Work out the finished part from the listing and answer in its coordinate system (mm). Give positions to 0.01 mm unless a question says otherwise; leave off trailing zeros. Loops run counter-clockwise (first coordinate to the right, second up) from the corner with the lowest first, then second, coordinate; pieces in that order, holes last. Notation, with made-up numbers: (23, 85) - (63, 85) arc R14 cw to (63, 111) - close; hole circle Ø11 at (-2, -35.75). An arc over 180 degrees is marked (long way). One line per item, written item: value.
from build123d import *

# Parameters (mm, degrees)
SKETCH_3_W          = 213
SKETCH_3_H          = 65.8
SKETCH_3_R          = 3
EXTRUDE_2_DEPTH     = 5
SKETCH_4_R          = 1.5
CUT_EXTRUDE_1_DEPTH = 5
SKETCH_5_R          = 1.5
CUT_EXTRUDE_2_DEPTH = 5
SKETCH_6_R          = 3
CUT_EXTRUDE_3_DEPTH = 10


with BuildPart() as part:
    # Sketch 3 → Extrude 2 (new body)
    with BuildSketch(Plane.XY):
        Rectangle(SKETCH_3_W, SKETCH_3_H)
        Circle(SKETCH_3_R, mode=Mode.SUBTRACT)
    extrude(amount=EXTRUDE_2_DEPTH)

    # Sketch 4 → Cut-Extrude 1 (cut)
    with BuildSketch(Plane.XY.offset(5)):
        with Locations((60, 12.1)):
            Circle(SKETCH_4_R)
        with Locations((60, -17.9)):
            Circle(SKETCH_4_R)
        with Locations(Location((-60, -17.9, 0), (0, 0, 180))):
            Circle(SKETCH_4_R)
        with Locations(Location((-60, 12.1, 0), (0, 0, 180))):
            Circle(SKETCH_4_R)
    extrude(amount=-CUT_EXTRUDE_1_DEPTH, mode=Mode.SUBTRACT)

    # Sketch 5 → Cut-Extrude 2 (cut)
    with BuildSketch(Plane.XY.offset(5)):
        with Locations((-100.5, 26)):
            Circle(SKETCH_5_R)
        with Locations((-100.5, 18)):
            Circle(SKETCH_5_R)
        with Locations((-100.5, -18)):
            Circle(SKETCH_5_R)
        with Locations((-100.5, -26)):
            Circle(SKETCH_5_R)
        with Locations((100.5, -4)):
            Circle(SKETCH_5_R)
        with Locations((100.5, 4)):
            Circle(SKETCH_5_R)
    extrude(amount=-CUT_EXTRUDE_2_DEPTH, mode=Mode.SUBTRACT)

    # Sketch 6 → Cut-Extrude 3 (cut)
    with BuildSketch(Plane.XY.offset(5)):
        with Locations((19, 0)):
            Circle(SKETCH_6_R)
        with Locations((-19, 0)):
            Circle(SKETCH_6_R)
    extrude(amount=-CUT_EXTRUDE_3_DEPTH, mode=Mode.SUBTRACT)


solid = part.part
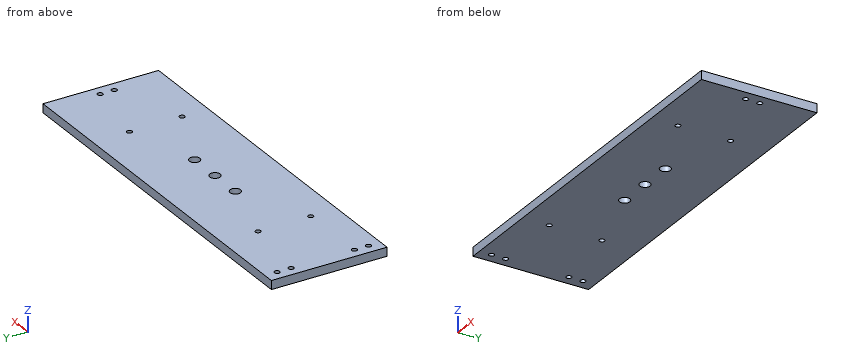
1. Section A-A (x = -19) is taken. Write down the section's boundary in (y, z).
Output:
outline: (-32.9, 0) - (-3, 0) - (-3, 5) - (-32.9, 5) - close; (3, 0) - (32.9, 0) - (32.9, 5) - (3, 5) - close
2. A flat-ended cylindrical pin translates along its axis: pin 1 Ø1.8 at (x, y) = (60, 12.1) entering from +Z. Find the tip coordinate at first contact, or state that the pin passes through.
Output:
pin 1: passes through
3. Find the intervals of material crossed by line 1 along Y through (x, z) = (-60, 2.55); line 2 along Y through (x, z) = (-100.5, 1.5); line 3 along Y through (x, z) = (100.5, 3.25), in increasing order.
Output:
line 1: y = -32.9 to -19.4, -16.4 to 10.6, 13.6 to 32.9
line 2: y = -32.9 to -27.5, -24.5 to -19.5, -16.5 to 16.5, 19.5 to 24.5, 27.5 to 32.9
line 3: y = -32.9 to -5.5, -2.5 to 2.5, 5.5 to 32.9
